```python
from build123d import *

# Parameters (mm, degrees)
F1_DEPTH  = 44
F2_R      = 4
F3_DEPTH  = 25
F4_DEPTH  = 25
F6_DEPTH  = 25
F5_R      = 4
F7_DEPTH  = 25
F8_R      = 3
F10_DEPTH = 25
F11_R     = 10
F12_R     = 7.25
F13_DEPTH = 25


with BuildPart() as f1:
    # F0 (on Front) → F1 (new body)
    with BuildSketch(Plane.XZ):
        Polygon((0, 74), (0, 0), (3, 0), (3, 70.2200388411), (33, 70.2200388411), (33, 0), (36, 0), (36, 74), align=None)
    extrude(amount=F1_DEPTH)

    # F2 (on face) → F3 (cut)
    with BuildSketch(Plane.YZ.offset(36)):
        with Locations((-34, 10)):
            Circle(F2_R)
    extrude(amount=-F3_DEPTH, mode=Mode.SUBTRACT)

    # F2 (on face) → F4 (cut)
    with BuildSketch(Plane.YZ.offset(36)):
        Polygon((0, 74), (-22, 0), (0, 0), align=None)
    extrude(amount=-F4_DEPTH, mode=Mode.SUBTRACT)

    # F5 (on face) → F6 (cut)
    with BuildSketch(Plane(origin=(0, 0, 0), x_dir=(0, -1, 0), z_dir=(-1, 0, 0))):
        Polygon((22, 0), (0, 74), (0, 0), align=None)
    extrude(amount=-F6_DEPTH, mode=Mode.SUBTRACT)

    # F5 (on face) → F7 (cut)
    with BuildSketch(Plane(origin=(0, 0, 0), x_dir=(0, -1, 0), z_dir=(-1, 0, 0))):
        with Locations((34, 10)):
            Circle(F5_R)
    extrude(amount=-F7_DEPTH, mode=Mode.SUBTRACT)

    # F8
    f8_edges = [f1.edges().sort_by_distance(p)[0] for p in [
        (36, -22, 74),
        (0, -22, 74),
        (33, -22.561886, 70.220039),
        (3, -22.561886, 70.220039),
    ]]
    fillet(f8_edges, radius=F8_R)

    # F9 (on face) → F10 (cut)
    with BuildSketch(Plane(origin=(0, 0, 0), x_dir=(0, -1, 0), z_dir=(-1, 0, 0))):
        with BuildLine():
            Line((32.75, 16), (32.75, 13.7996710384))
            ThreePointArc((32.75, 13.7996710384), (34, 14), (35.25, 13.7996710384))
            Line((35.25, 13.7996710384), (35.25, 16))
            Line((35.25, 16), (32.75, 16))
        make_face()
    extrude(amount=-F10_DEPTH, mode=Mode.SUBTRACT)

    # F11
    f11_edges = [f1.edges().sort_by_distance(p)[0] for p in [
        (1.5, -22, 0),
        (1.5, -44, 0),
        (34.5, -44, 0),
        (34.5, -22, 0),
    ]]
    fillet(f11_edges, radius=F11_R)

    # F12 (on face) → F13 (cut)
    with BuildSketch(Plane.XY.offset(74)):
        with Locations((18, -22)):
            Circle(F12_R)
    extrude(amount=-F13_DEPTH, mode=Mode.SUBTRACT)


solid = f1.part
```
Geometry: final body of the model. Coordinates: model frame, mm. A direction names the side the tool comes from. Round coordinates to 2 decimals unless told otherwise and drop trailing zeros. Order: outer loops, then holes, each group sorted by start corner. A loop starts at its lowest first (then second) coordinate and runs counter-clockwise, first axis right, second up. Notation, with made-up numbers: (-40, 50) -> (2, 50) arc R14 ccw to (2, 76) -> close; hole circle Ø1 at (-23, 41). An arc over 180 degrees is marked (long way). Write each question's results on one line, items separated by ' | '.
Q1. Access query for faces 4 (the face through (0.86, -22.31, 73.1)), 5 (the face through (33, -27, 42)). Directions: +Z, -Z, +X, -X, +Y, -Y. A direction counts if a zero-diameter tool reaches every point of the face in a straight line with its end or side. Return the directions, or none.
Response values:
face 4: +Z, -X, +Y, -Y | face 5: -Z, +Y, -Y
Q2. Ray query, line 1 along X through (y, z) = (-35.5, 50); line 2 along Z through (x, y) = (28.5, -7); line 3 along Y through (x, z) = (18, 72.55). Return the intervals inside material, ascending.
Response values:
line 1: 0 to 3, 33 to 36 | line 2: 70.22 to 74 | line 3: -44 to -29.25, -14.75 to -0.43
Q3. Section query B-B (y = -22). Output: boundary loops of the cut face in (x, z), and give its area (3 significant figures).
Response values:
outline: (0, 3.34) -> (3, 3.34) -> (3, 67.22) arc R3 cw to (6, 70.22) -> (10.75, 70.22) -> (10.75, 74) -> (3, 74) arc R3 ccw to (0, 71) -> close; (25.25, 70.22) -> (30, 70.22) arc R3 cw to (33, 67.22) -> (33, 3.34) -> (36, 3.34) -> (36, 71) arc R3 ccw to (33, 74) -> (25.25, 74) -> close | area: 483 mm²
Q4. Pin query (flat end, axial travel): pin 1 Ø5 at (x, y) = (10, -30.5) entering from -Z; pin 2 Ø1.1 at (x, z) = (1.5, 15) entering from +Y. Return the tip coordinate at first contact, or that it passes through.
Response values:
pin 1: z = 70.22 | pin 2: y = -17.38
Q5. Section query D-D (y = -40). Output: boundary loops of the cut face in (x, z).
Response values:
outline: (0, 2) -> (3, 2) -> (3, 67.22) arc R3 cw to (6, 70.22) -> (30, 70.22) arc R3 cw to (33, 67.22) -> (33, 2) -> (36, 2) -> (36, 71) arc R3 ccw to (33, 74) -> (3, 74) arc R3 ccw to (0, 71) -> close
Q6. Pull-direction query (Z, two-part tool) for faces 1 (the face through (36, -27, 43)), 2 (the face through (32.1, -22.86, 69.36)), 3 (the face through (1, -35.25, 15)); classes: released by +Z, released by -Z, zero draft, split by the parting line, or undercut.
Response values:
face 1: zero draft | face 2: released by -Z | face 3: undercut
Q7. Section query A-A (x = 18). Output: boundary loops of the cut face in (y, z).
Response values:
outline: (-44, 70.22) -> (-29.25, 70.22) -> (-29.25, 74) -> (-44, 74) -> close; (-14.75, 70.22) -> (-1.12, 70.22) -> (0, 74) -> (-14.75, 74) -> close
Q8. Section query C-C (z = 12). Output: boundary loops of the cut face in (x, y).
Response values:
outline: (0, -44) -> (3, -44) -> (3, -37.46) -> (0, -37.46) -> close; (0, -30.54) -> (3, -30.54) -> (3, -18.43) -> (0, -18.43) -> close; (33, -44) -> (36, -44) -> (36, -37.46) -> (33, -37.46) -> close; (33, -30.54) -> (36, -30.54) -> (36, -18.43) -> (33, -18.43) -> close
